from build123d import *

# Parameters (mm, degrees)
F0_W     = 55.175
F0_H     = 176
F1_DEPTH = 5


with BuildPart() as f1:
    # F0 (on Top) → F1 (new body)
    with BuildSketch(Plane.XY):
        Rectangle(F0_W, F0_H)
        with BuildLine():
            ThreePointArc((-24.5625, -43.303427), (-24.5625, -40.475), (-21.734073, -40.475))
            Line((-21.734073, -40.475), (-7.340927, -40.475))
            ThreePointArc((-7.340927, -40.475), (-4.5125, -40.475), (-4.5125, -43.303427))
            Line((-4.5125, -43.303427), (-4.5125, -55.775))
            Line((-4.5125, -55.775), (-4.5125, -78.696573))
            ThreePointArc((-4.5125, -78.696573), (-4.5125, -81.525), (-7.340927, -81.525))
            Line((-7.340927, -81.525), (-21.734073, -81.525))
            ThreePointArc((-21.734073, -81.525), (-24.5625, -81.525), (-24.5625, -78.696573))
            Line((-24.5625, -78.696573), (-24.5625, -55.775))
            Line((-24.5625, -55.775), (-24.5625, -43.303427))
        make_face(mode=Mode.SUBTRACT)
        with BuildLine():
            Line((-24.5625, 43.303427), (-24.5625, 55.775))
            Line((-24.5625, 55.775), (-24.5625, 78.696573))
            ThreePointArc((-24.5625, 78.696573), (-24.5625, 81.525), (-21.734073, 81.525))
            Line((-21.734073, 81.525), (-7.340927, 81.525))
            ThreePointArc((-7.340927, 81.525), (-4.5125, 81.525), (-4.5125, 78.696573))
            Line((-4.5125, 78.696573), (-4.5125, 55.775))
            Line((-4.5125, 55.775), (-4.5125, 43.303427))
            ThreePointArc((-4.5125, 43.303427), (-4.5125, 40.475), (-7.340927, 40.475))
            Line((-7.340927, 40.475), (-21.734073, 40.475))
            ThreePointArc((-21.734073, 40.475), (-24.5625, 40.475), (-24.5625, 43.303427))
        make_face(mode=Mode.SUBTRACT)
    extrude(amount=F1_DEPTH)


solid = f1.part
Verification items for the finished model (mm, model axes). A direction names the side the tool comes from. Round coordinates to 2 decimals unless told otherwise and drop trailing zeros. Loops run counter-clockwise (first coordinate to the right, second up) from the corner with the lowest first, then second, coordinate; pieces in that order, holes last. Notation, with made-up numbers: (-33.5, 0) - (-9.5, 0) arc R15 ccw to (-9.5, 15) - close; hole circle Ø8 at (50, -30). An arc over 180 degrees is marked (long way). Answer in a Markdown table with one row per item. Add a question column.
Q1. Release check for a two-part mould opening along Y. For faces 3 (the face through (27.588, -1, 2)), 4 (the face through (-24.562, -61, 2)), 5 (the face through (-24.531, 40.444, 2.465)), 6 (the face through (0, -88, 2)) record: pulls with the +Y half, pulls with the -Y half, needs draft (parallel to the pull), parting line crosses it, or undercut.
Q2. Section check C-C on z = 2.25. Enter the section's corners in (x, y) (1 decimal), plus the area to 3 significant figures.
Q3. Section check B-B on y = -57.5. Enter the section's corners in (x, z), plus the area to 3 significant figures.
Q4. Section check A-A on x = -10.5. Enter the section's corners in (y, z) (3 decimals).
Q5. Tool access check on faces 1 (the face through (0, 1, 0)), 2 (the face through (-15, 81.525, 2)). Record the directions out of +Z, -Z, +X, -X, +Y, -Y that give a thin tool (end or side, any length) a straight path to the whole face; none if there is none.
Q6. Material ranges on line 1 (Y direction, x = -20.5, z = 4.2) (3 decimals); line 2 (X direction, y = -44, z = 0.75); line 3 (Y direction, x = -5.5, z = 1.6), recorded low to high.
Found:
| question | item | result |
|---|---|---|
| 1 | face 3 | needs draft |
| 1 | face 4 | undercut |
| 1 | face 5 | undercut |
| 1 | face 6 | pulls with the -Y half |
| 2 | outline | (-27.6, -88) - (27.6, -88) - (27.6, 88) - (-27.6, 88) - close; hole (-24.6, -78.7) arc R2 ccw to (-21.7, -81.5) - (-7.3, -81.5) arc R2 ccw to (-4.5, -78.7) - (-4.5, -43.3) arc R2 ccw to (-7.3, -40.5) - (-21.7, -40.5) arc R2 ccw to (-24.6, -43.3) - close; hole (-24.6, 43.3) arc R2 ccw to (-21.7, 40.5) - (-7.3, 40.5) arc R2 ccw to (-4.5, 43.3) - (-4.5, 78.7) arc R2 ccw to (-7.3, 81.5) - (-21.7, 81.5) arc R2 ccw to (-24.6, 78.7) - close |
| 2 | area | 8,050 mm² |
| 3 | outline | (-27.59, 0) - (-24.56, 0) - (-24.56, 5) - (-27.59, 5) - close; (-4.51, 0) - (27.59, 0) - (27.59, 5) - (-4.51, 5) - close |
| 3 | area | 176 mm² |
| 4 | outline | (-88, 0) - (-81.525, 0) - (-81.525, 5) - (-88, 5) - close; (-40.475, 0) - (40.475, 0) - (40.475, 5) - (-40.475, 5) - close; (81.525, 0) - (88, 0) - (88, 5) - (81.525, 5) - close |
| 5 | face 1 | -Z, +X, -X, +Y, -Y |
| 5 | face 2 | +Z, -Z |
| 6 | line 1 | y = -88 to -81.525, -40.475 to 40.475, 81.525 to 88 |
| 6 | line 2 | x = -27.59 to -24.56, -4.51 to 27.59 |
| 6 | line 3 | y = -88 to -82.06, -39.94 to 39.94, 82.06 to 88 |
